Part model, mm, in its own coordinate system. A direction names the side the tool comes from. Round coordinates to 2 decimals unless told otherwise and drop trailing zeros. Write each loop counter-clockwise with the first axis right and the second up, starting at its lowest first coordinate (ties: lowest second). Pieces come first, ordered by that corner, then holes. Notation, with made-up numbers: M 30,-37.5 L 59,-37.5 A15 ccw 59,-17.5 Z; hole C -24,50.5 d2. An arc over 180 degrees is marked long. One line per question, with ' | ' between items. Start each with the question number.
1) Tool access for faces 4 (the face through (0.64, 2.58, 4.05)), 5 (the face through (-46, -1.13, -3.13)): list every direction of +Z, -Z, +X, -X, +Y, -Y with a clear straight run to the whole face (end or side of a thin tool).
2) Saw through at A-A (x = 33.5). List the corners of the cut face in (y, z).
3) Drop flat-ended pins along their axis: pin 1 Ø2 at (x, y) = (-15.5, 2.5) entering from -Z; pin 2 Ø4 at (x, y) = (-12.5, -3.5) entering from +Z. Give the stop position or say it passes through.
4) Mould opens along Z. For faces 1 (the face through (37.984, -2.435, 0.767)), 2 (the face through (-51.42, 0.69, -3.1)), 3 (the face through (-57, 0, 0)) say: pulls with the +Z half, pulls with the -Z half, needs draft (parallel to the pull), parting line crosses it, or undercut.
5) Saw through at B-B (x = -15). List the corners of the cut face in (y, z).
6) Wall check: probe 1 along Z at (x, y) = (38, 0); probe 2 along X at (y, z) = (-1.25, -3.5); probe 3 along Z at (x, y) = (41, 2.25). Give the ranges that are in metal, low to high. Write a range as [from, to].
```python
from build123d import *

# Parameters (mm, degrees)
F0_R     = 4.8
F1_DEPTH = 46
F3_D     = 5.1054
F3_DEPTH = 15.81
F3_TIP   = 1.5338169022
F4_R     = 3.175
F5_DEPTH = 11


with BuildPart() as f1:
    # F0 (on Right) → F1 (new body, symmetric)
    with BuildSketch(Plane.YZ):
        Circle(F0_R)
    extrude(amount=F1_DEPTH, both=True)

    # F3
    with Locations(Plane.YZ.offset(46)):
        with Locations((0, 0)):
            Hole(F3_D / 2, depth=F3_DEPTH)
            with Locations((0, 0, -(F3_DEPTH + F3_TIP / 2))):  # 118° drill point
                Cone(0, F3_D / 2, F3_TIP, mode=Mode.SUBTRACT)

    # F4 (on face) → F5 (join)
    with BuildSketch(Plane(origin=(-46, 0, 0), x_dir=(0, -1, 0), z_dir=(-1, 0, 0))):
        Circle(F4_R)
    extrude(amount=F5_DEPTH)


solid = f1.part
```
Answer key:
1) face 4: +X, -X | face 5: -X
2) outline: C 0,0 d9.6; hole C 0,0 d5.11
3) pin 1: stops at z = -4.56 | pin 2: stops at z = 4.56
4) face 1: undercut | face 2: parting line crosses it | face 3: needs draft
5) outline: C 0,0 d9.6
6) probe 1: z = [-4.8, -2.55], [2.55, 4.8] | probe 2: x = [-46, 46] | probe 3: z = [-4.24, -1.21], [1.21, 4.24]
